```python
from build123d import *

# Parameters (mm, degrees)
SKETCH1_R           = 32.5
SKETCH1_R_2         = 1
BOSS_EXTRUDE1_DEPTH = 3
SKETCH2_R           = 22.5
SKETCH2_R_2         = 2
CUT_EXTRUDE1_DEPTH  = 47.059743812


with BuildPart() as part:
    # Sketch1 → Boss-Extrude1 (new body)
    with BuildSketch(Plane(origin=(0, 0, 0), x_dir=(1, 0, 0), z_dir=(0, 1, 0))):
        with Locations(Location((0, 0, 0), (0, 0, 270))):
            Circle(SKETCH1_R)
        with Locations(Location((0, 27, 0), (0, 0, 270))):
            Circle(SKETCH1_R_2, mode=Mode.SUBTRACT)
        with Locations(Location((23.382685902, 13.5, 0), (0, 0, 270))):
            Circle(SKETCH1_R_2, mode=Mode.SUBTRACT)
        with Locations(Location((23.382685902, -13.5, 0), (0, 0, 270))):
            Circle(SKETCH1_R_2, mode=Mode.SUBTRACT)
        with Locations(Location((0, -27, 0), (0, 0, 270))):
            Circle(SKETCH1_R_2, mode=Mode.SUBTRACT)
        with Locations(Location((-23.382685902, -13.5, 0), (0, 0, 270))):
            Circle(SKETCH1_R_2, mode=Mode.SUBTRACT)
        with Locations(Location((-23.382685902, 13.5, 0), (0, 0, 270))):
            Circle(SKETCH1_R_2, mode=Mode.SUBTRACT)
    extrude(amount=BOSS_EXTRUDE1_DEPTH)

    # Sketch2 → Cut-Extrude1 (cut, through all)
    with BuildSketch(Plane(origin=(0, 3, 0), x_dir=(1, 0, 0), z_dir=(0, 1, 0))):
        with Locations(Location((0, 0, 0), (0, 0, 270))):
            Circle(SKETCH2_R)
        with Locations(Location((-13.5, 23.382685902, 0), (0, 0, 270))):
            Circle(SKETCH2_R_2)
        with Locations(Location((13.5, 23.382685902, 0), (0, 0, 270))):
            Circle(SKETCH2_R_2)
        with Locations(Location((27, 0, 0), (0, 0, 270))):
            Circle(SKETCH2_R_2)
        with Locations(Location((13.5, -23.382685902, 0), (0, 0, 270))):
            Circle(SKETCH2_R_2)
        with Locations(Location((-13.5, -23.382685902, 0), (0, 0, 270))):
            Circle(SKETCH2_R_2)
        with Locations(Location((-27, 0, 0), (0, 0, 270))):
            Circle(SKETCH2_R_2)
    extrude(amount=-CUT_EXTRUDE1_DEPTH, mode=Mode.SUBTRACT)


solid = part.part
```
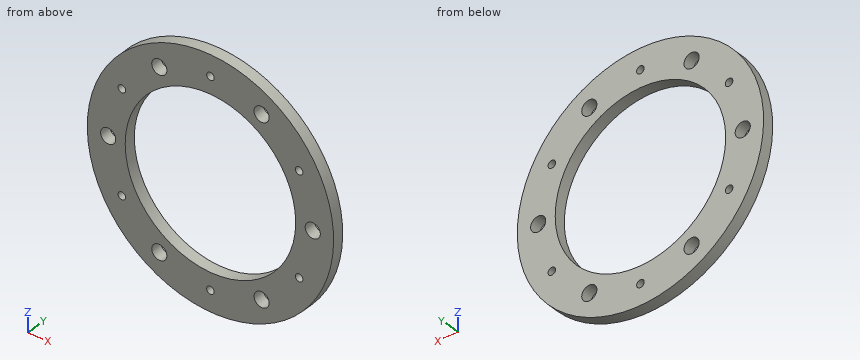
Design review of the part built by this model. Coordinates are the model's own, in mm. Give positions to 0.01 mm unless a question says otherwise; leave off trailing zeros. Write each loop counter-clockwise with the first axis right and the second up, starting at its lowest first coordinate (ties: lowest second). Pieces come first, ordered by that corner, then holes. Notation, with made-up numbers: (-19.5, 89.25) -> (36.5, 89.25) arc R28 ccw to (36.5, 119.25) -> close; hole circle Ø9 at (74.25, 50.25). An arc over 180 degrees is marked (long way). Answer in a Markdown table with one row per item.
(1) Consider section A-A (z = 0). State the section outline as (x, y) points, then the cut area to 3 significant figures.
Results:
| item | result |
|---|---|
| outline | (-32.5, 0) -> (-29, 0) -> (-29, 3) -> (-32.5, 3) -> close; (-25, 0) -> (-22.5, 0) -> (-22.5, 3) -> (-25, 3) -> close; (22.5, 0) -> (25, 0) -> (25, 3) -> (22.5, 3) -> close; (29, 0) -> (32.5, 0) -> (32.5, 3) -> (29, 3) -> close |
| area | 36.0 mm2 |
(2) Clearance check with flat-ended pins moving along their axes: pin 1 (2.5 mm diameter, centred on x = -27, z = 0, fed in from -Y); pin 2 (1.5 mm diameter, centred on x = 22.5, y = 2, fed in from -Z). State where each tip first meets the part, or that it passes through.
Results:
| item | result |
|---|---|
| pin 1 | through |
| pin 2 | z = -24.15 |
(3) To check wall thickness, follow probe 1 along X at (y, z) = (1.2, 0); probe 2 along X at (y, z) = (1.15, 13.5); probe 3 along X at (y, z) = (1.5, 23.5). State the ranges of each line that lie inside material, in increasing order.
Results:
| item | result |
|---|---|
| probe 1 | -32.5 to -29, -25 to -22.5, 22.5 to 25, 29 to 32.5 |
| probe 2 | -29.56 to -24.38, -22.38 to -18, 18 to 22.38, 24.38 to 29.56 |
| probe 3 | -22.45 to -15.5, -11.5 to 11.5, 15.5 to 22.45 |
(4) Consider section C-C (x = -21). State the section outline as (y, z) points, then the cut area to 3 significant figures.
Results:
| item | result |
|---|---|
| outline | (0, -24.8) -> (3, -24.8) -> (3, -8.08) -> (0, -8.08) -> close; (0, 8.08) -> (3, 8.08) -> (3, 24.8) -> (0, 24.8) -> close |
| area | 100 mm2 |
(5) Consider section D-D (y = 1.7). Count the separate pieces of the cut face and the enclosed holes in it, then the cut area to 3 significant figures.
Results:
| item | result |
|---|---|
| separate pieces | 1 |
| enclosed holes | 13 |
| area | 1,630 mm2 |
(6) Consider section B-B (x = 0). State the section outline as (y, z) points, then the cut area to 3 significant figures.
Results:
| item | result |
|---|---|
| outline | (0, -32.5) -> (3, -32.5) -> (3, -28) -> (0, -28) -> close; (0, -26) -> (3, -26) -> (3, -22.5) -> (0, -22.5) -> close; (0, 22.5) -> (3, 22.5) -> (3, 26) -> (0, 26) -> close; (0, 28) -> (3, 28) -> (3, 32.5) -> (0, 32.5) -> close |
| area | 48.0 mm2 |
